from build123d import *

# Parameters (mm, degrees)
SKETCH1_W                       = 75
SKETCH1_H                       = 187.5
SKETCH1_W_2                     = 55
SKETCH1_H_2                     = 167.5
BOSS_EXTRUDE1_DEPTH             = 59
TAP_DRILL_FOR_M5X0_8_TAP2_D     = 4.2
TAP_DRILL_FOR_M5X0_8_TAP2_DEPTH = 10
TAP_DRILL_FOR_M5X0_8_TAP3_D     = 4.2
TAP_DRILL_FOR_M5X0_8_TAP3_DEPTH = 10
TAP_DRILL_FOR_M5X0_8_TAP3_TIP   = 1.2618073
SKETCH13_W                      = 15
SKETCH13_H                      = 6.35
SKETCH13_H_2                    = 5
BOSS_EXTRUDE2_DEPTH             = 55
SKETCH14_W                      = 6.35
SKETCH14_H                      = 10.3
BOSS_EXTRUDE3_DEPTH             = 25
TAP_DRILL_FOR_M2_5X0_45_TAP1_D  = 2.05
TAP_DRILL_FOR_M3X0_5_TAP1_D     = 2.5
TAP_DRILL_FOR_M3X0_5_TAP1_DEPTH = 10


with BuildPart() as part:
    # Sketch1 → Boss-Extrude1 (new body)
    with BuildSketch(Plane.XY):
        with Locations((37.5, 93.75)):
            Rectangle(SKETCH1_W, SKETCH1_H)
        with Locations((37.5, 93.75)):
            Rectangle(SKETCH1_W_2, SKETCH1_H_2, mode=Mode.SUBTRACT)
    extrude(amount=-BOSS_EXTRUDE1_DEPTH)

    # Tap Drill for M5x0.8 Tap2
    with Locations(Plane(origin=(0, 10, 0), x_dir=(1, 0, 0), z_dir=(0, 1, 0))):
        with Locations((37.5, 29.5)):
            Hole(TAP_DRILL_FOR_M5X0_8_TAP2_D / 2, depth=TAP_DRILL_FOR_M5X0_8_TAP2_DEPTH)

    # Tap Drill for M5x0.8 Tap3
    with Locations(Plane(origin=(0, 187.5, 0), x_dir=(1, 0, 0), z_dir=(0, 1, 0))):
        with Locations((37.5, 29.5)):
            Hole(TAP_DRILL_FOR_M5X0_8_TAP3_D / 2, depth=TAP_DRILL_FOR_M5X0_8_TAP3_DEPTH)
            with Locations((0, 0, -(TAP_DRILL_FOR_M5X0_8_TAP3_DEPTH + TAP_DRILL_FOR_M5X0_8_TAP3_TIP / 2))):  # 118° drill point
                Cone(0, TAP_DRILL_FOR_M5X0_8_TAP3_D / 2, TAP_DRILL_FOR_M5X0_8_TAP3_TIP, mode=Mode.SUBTRACT)

    # Sketch13 → Boss-Extrude2 (add)
    with BuildSketch(Plane(origin=(0, 10, 0), x_dir=(1, 0, 0), z_dir=(0, 1, 0))):
        with Locations((57.5, 35.925)):
            Rectangle(SKETCH13_W, SKETCH13_H)
        with Locations((17.5, 35.925)):
            Rectangle(SKETCH13_W, SKETCH13_H)
        with Locations((17.5, 8.75)):
            Rectangle(SKETCH13_W, SKETCH13_H_2)
        with Locations((57.5, 8.75)):
            Rectangle(SKETCH13_W, SKETCH13_H_2)
    extrude(amount=BOSS_EXTRUDE2_DEPTH)

    # Sketch14 → Boss-Extrude3 (add)
    with BuildSketch(Plane.ZY.offset(-50)):
        with Locations((-35.925, 59.85)):
            Rectangle(SKETCH14_W, SKETCH14_H)
    extrude(amount=BOSS_EXTRUDE3_DEPTH)

    # Tap Drill for M2.5x0.45 Tap1 (through all)
    with Locations(Plane(origin=(0, 0, -39.1), x_dir=(-1, 0, 0), z_dir=(0, 0, -1))):
        with Locations((-46, 57.8), (-52.5, 51.5), (-52.5, 34.5), (-52.5, 17.5), (-22.5, 17.5), (-22.5, 34.5), (-22.5, 51.5), (-29, 57.8)):
            Hole(TAP_DRILL_FOR_M2_5X0_45_TAP1_D / 2)

    # Tap Drill for M3x0.5 Tap1
    with Locations(Plane(origin=(0, 10, 0), x_dir=(1, 0, 0), z_dir=(0, 1, 0))):
        with Locations((13, 3.125), (62, 3.125), (60, 53), (15, 53)):
            Hole(TAP_DRILL_FOR_M3X0_5_TAP1_D / 2, depth=TAP_DRILL_FOR_M3X0_5_TAP1_DEPTH)


solid = part.part
Build history of the part. All positions in model axes, mm. A direction names the side the tool comes from. Round coordinates to 2 decimals unless told otherwise and drop trailing zeros. Loops run counter-clockwise (first coordinate to the right, second up) from the corner with the lowest first, then second, coordinate; pieces in that order, holes last. Notation, with made-up numbers: (16.25, 87.5) -> (24.25, 87.5) arc R25 ccw to (24.25, 101.5) -> close; hole circle Ø4 at (28, -37.75). An arc over 180 degrees is marked (long way). One line per item, written item: value. Start each with the question number.
Q1. Cut at A-A on z = -29.5. List the corners of the cut face in (x, y), plus the area to 3 significant figures.
Q2. Two-plate mould, pull along X, no slides. Class faces 4 (the face through (9.5, 115, -59)), 5 (the face through (75, 92, -29)), 6 (the face through (57, 37, -11.25)): released by +X, released by -X, zero draft, split by the parting line, or undercut.
Q3. Probe line 1 along X through (y, z) = (5.5, -53); line 2 along Y through (x, z) = (52.5, -7.55) (3 decimals); line 3 along X through (y, z) = (165.5, -31). List the from-to ranges inside material, lowest first.
Q4. Cut at C-C on y = 127. List the corners of the cut face in (x, z).
Q5. Cut at B-B on x = 56. List the corners of the cut face in (y, z).
Q6. Cut at D-D on z = -19.5. List the corners of the cut face in (x, y), plus the area to 3 significant figures.
Q7. 3-axis set-ups, long thin cutter, end or side, ignore diameter. For faces 1 (the face through (37, 10, -36)), 2 (the face through (57, 37, -6.25)), 3 (the face through (25, 32, -36)): which of +Z, -Z, +X, -X, +Y, -Y reach the whole face in a straight line?
Computed:
1. outline: (0, 0) -> (35.4, 0) -> (35.4, 10) -> (10, 10) -> (10, 177.5) -> (35.4, 177.5) -> (35.4, 187.5) -> (0, 187.5) -> close; (39.6, 0) -> (75, 0) -> (75, 187.5) -> (39.6, 187.5) -> (39.6, 177.5) -> (65, 177.5) -> (65, 10) -> (39.6, 10) -> close
1. area: 4,770 mm²
2. face 4: zero draft
2. face 5: released by +X
2. face 6: undercut
3. line 1: 0 to 13.75, 16.25 to 58.75, 61.25 to 75
3. line 2: 0 to 16.475, 18.525 to 33.475, 35.525 to 50.475, 52.525 to 65, 177.5 to 187.5
3. line 3: 0 to 10, 65 to 75
4. outline: (0, -59) -> (10, -59) -> (10, 0) -> (0, 0) -> close; (65, -59) -> (75, -59) -> (75, 0) -> (65, 0) -> close
5. outline: (0, -59) -> (10, -59) -> (10, -39.1) -> (65, -39.1) -> (65, -32.75) -> (10, -32.75) -> (10, -11.25) -> (65, -11.25) -> (65, -6.25) -> (10, -6.25) -> (10, 0) -> (0, 0) -> close; (177.5, -59) -> (187.5, -59) -> (187.5, 0) -> (177.5, 0) -> close
6. outline: (0, 0) -> (75, 0) -> (75, 187.5) -> (0, 187.5) -> close; hole (10, 10) -> (65, 10) -> (65, 177.5) -> (10, 177.5) -> close
6. area: 4,850 mm²
7. face 1: none
7. face 2: +Z
7. face 3: +Z, -Z
